Read the model definition and answer for the solid it produces. Units are mm, in the model's axes. A direction names the side the tool comes from. Coordinates: 2 decimals unless noted, no trailing zeros. Order: outer loops, then holes, each group sorted by start corner. A loop starts at its lowest first (then second) coordinate and runs counter-clockwise, first axis right, second up. Notation, with made-up numbers: M 50,57.25 L 83,57.25 A19 cw 83,80.25 Z; hole C 89.5,-27.5 d8. An arc over 180 degrees is marked long. Use a Markdown table: item, result. Add a question column.
1) Each of these flat-tipped pins is pushed along its axis until it touches: pin 1 Ø1 at (y, z) = (100, -25) entering from -X; pin 2 Ø0.9 at (x, y) = (9.5, 155.5) entering from +Z; pin 3 Ø5.5 at (x, y) = (143, 67) entering from +Z; pin 4 Ø2.5 at (x, y) = (149.5, 4) entering from -Z. Where does it stop, or does it pass through?
2) Find section A-A on x = 69.5. Write down the section's boundary in (y, z).
3) Find section B-B on y = 98. Write down the section's boundary in (x, z), plus the area to 3 significant figures.
4) For faces 4 (the face through (153.006, 153, -7)), 5 (the face through (151, 5, -13)), 6 (the face through (10.37, 78, -6)), 7 (the face through (5, 124, -3.5)), determine the directions among +Z, -Z, +X, -X, +Y, -Y from which every point of the face is accessible in a straight line to the end or side of a thin tool.
5) Find section C-C on z = -27.25. Write down the section's boundary in (x, y).
6) Find the intervals of material crossed by probe 1 along Y at (x, z) = (49, -3); probe 2 along Y at (x, z) = (3.75, -2.15) (3 decimals); probe 3 along X at (y, z) = (155, -1.8), in increasing order. Write a range as [from, to].
7) The mould has two halves that part along Y. Classify faces 1 (the face through (81, 148.38, -6)), 2 (the face through (2.406, 2.281, -7.768)), 3 (the face through (153.006, 5, -7)): released by +Y, released by -Y, zero draft, split by the parting line, or undercut.
from build123d import *

# Parameters (mm, degrees)
EXTRUDE_1_DEPTH      = 30
SKETCH_2_R           = 1.5
CUT_EXTRUDE_1_DEPTH  = 5
CUT_EXTRUDE_4_DEPTH  = 307
SKETCH_3_W           = 285.26
SKETCH_3_H           = 138.01
CUT_EXTRUDE_5_DEPTH  = 13
SKETCH_12_W          = 40
SKETCH_12_H          = 50
CUT_EXTRUDE_7_DEPTH  = 3
CUT_EXTRUDE_7_DRAFT  = -30
SKETCH_9_W           = 100
SKETCH_9_H           = 80
CUT_EXTRUDE_8_DEPTH  = 3
CUT_EXTRUDE_8_DRAFT  = -30
CUT_EXTRUDE_9_DEPTH  = 11
FILLET_1_R           = 2
CUT_EXTRUDE_10_DEPTH = 11
FILLET_2_R           = 2
FILLET_3_R           = 2
FILLET_4_R           = 2
CUT_EXTRUDE_11_DEPTH = 5


with BuildPart() as part:
    # Model → 凸台-拉伸1 (new body)
    with BuildSketch(Plane.XY):
        with BuildLine():
            Line((0, 11), (0, 150.75))
            ThreePointArc((0, 150.75), (2.343145751, 156.406854249), (8, 158.75))
            Line((8, 158.75), (298.011203897, 158.75))
            ThreePointArc((298.011203897, 158.75), (303.664092807, 156.410816811), (306.011196041, 150.761211743))
            Line((306.011196041, 150.761211743), (306.207051361, 11.011211743))
            Line((306.207051361, 11.011211743), (306.207051361, 8))
            ThreePointArc((306.207051361, 8), (303.863905611, 2.343145751), (298.207051361, 0))
            Line((298.207051361, 0), (8, 0))
            ThreePointArc((8, 0), (2.343145751, 2.343145751), (0, 8))
            Line((0, 8), (0, 11))
        make_face()
    extrude(amount=-EXTRUDE_1_DEPTH)

    # 草图2 → 切除-拉伸1 (cut)
    with BuildSketch(Plane.XY):
        with Locations((105.108569936, 3.75)):
            Circle(SKETCH_2_R)
        with Locations((9.108569936, 3.75)):
            Circle(SKETCH_2_R)
        with Locations((201.10846029, 3.817270412)):
            Circle(SKETCH_2_R)
        with Locations((297.108366012, 3.951811323)):
            Circle(SKETCH_2_R)
        with Locations((105.108569936, 155)):
            Circle(SKETCH_2_R)
        with Locations((9.108569936, 155)):
            Circle(SKETCH_2_R)
        with Locations((201.10846029, 154.932729588)):
            Circle(SKETCH_2_R)
        with Locations((297.108366012, 154.798188677)):
            Circle(SKETCH_2_R)
        with Locations((3.75, 109.375)):
            Circle(SKETCH_2_R)
        with Locations((3.75, 49.375)):
            Circle(SKETCH_2_R)
        with Locations((302.318900647, 109.584217456)):
            Circle(SKETCH_2_R)
        with Locations((302.402988717, 49.58427638)):
            Circle(SKETCH_2_R)
    extrude(amount=-CUT_EXTRUDE_1_DEPTH, mode=Mode.SUBTRACT)

    # 草图6 → 切除-拉伸4 (cut)
    with BuildSketch(Plane.ZY):
        Polygon((-30, 158.75), (-30, 0), (-15, 0), align=None)
    extrude(amount=-CUT_EXTRUDE_4_DEPTH, mode=Mode.SUBTRACT)

    # 草图3 → 切除-拉伸5 (cut)
    with BuildSketch(Plane.XY):
        with Locations((153, 79.375)):
            Rectangle(SKETCH_3_W, SKETCH_3_H)
    extrude(amount=-CUT_EXTRUDE_5_DEPTH, mode=Mode.SUBTRACT)


with BuildPart() as cut_extrude_7_tool:
    # 草图12 → 切除-拉伸7 (with draft: the straight prism first)
    with BuildSketch(Plane.XY.offset(-13)):
        with Locations((153, 70.37)):
            Rectangle(SKETCH_12_W, SKETCH_12_H)
    extrude(amount=-CUT_EXTRUDE_7_DEPTH)
    # 切除-拉伸7: the draft: its side faces are tilted about the plane it starts from
    cut_extrude_7_sides = [cut_extrude_7_tool.faces().sort_by_distance(p)[0] for p in [
        (153, 45.37, -14.5),
        (173, 70.37, -14.5),
        (153, 95.37, -14.5),
        (133, 70.37, -14.5),
    ]]
    draft(cut_extrude_7_sides, Plane.XY.offset(-13), CUT_EXTRUDE_7_DRAFT)


with BuildPart() as part_1:
    add(part.part)

    # 切除-拉伸7: cut by cut_extrude_7_tool
    add(cut_extrude_7_tool.part, mode=Mode.SUBTRACT)


with BuildPart() as cut_extrude_8_tool:
    # 草图9 → 切除-拉伸8 (with draft: the straight prism first)
    with BuildSketch(Plane.XY.offset(-13)):
        with Locations((75.37, 88.38)):
            Rectangle(SKETCH_9_W, SKETCH_9_H)
    extrude(amount=-CUT_EXTRUDE_8_DEPTH)
    # 切除-拉伸8: the draft: its side faces are tilted about the plane it starts from
    cut_extrude_8_sides = [cut_extrude_8_tool.faces().sort_by_distance(p)[0] for p in [
        (25.37, 88.38, -14.5),
        (75.37, 48.38, -14.5),
        (125.37, 88.38, -14.5),
        (75.37, 128.38, -14.5),
    ]]
    draft(cut_extrude_8_sides, Plane.XY.offset(-13), CUT_EXTRUDE_8_DRAFT)


with BuildPart() as part_2:
    add(part_1.part)

    # 切除-拉伸8: cut by cut_extrude_8_tool
    add(cut_extrude_8_tool.part, mode=Mode.SUBTRACT)

    # 草图14 → 切除-拉伸9 (cut)
    with BuildSketch(Plane.ZY):
        with BuildLine():
            Line((-5.9, 129.38), (-6.1, 129.38))
            ThreePointArc((-6.1, 129.38), (-7.797056275, 128.677056275), (-8.5, 126.98))
            Line((-8.5, 126.98), (-8.5, 120.78))
            ThreePointArc((-8.5, 120.78), (-7.797056275, 119.082943725), (-6.1, 118.38))
            Line((-6.1, 118.38), (-5.9, 118.38))
            ThreePointArc((-5.9, 118.38), (-4.202943725, 119.082943725), (-3.5, 120.78))
            Line((-3.5, 120.78), (-3.5, 126.98))
            ThreePointArc((-3.5, 126.98), (-4.202943725, 128.677056275), (-5.9, 129.38))
        make_face()
    extrude(amount=-CUT_EXTRUDE_9_DEPTH, mode=Mode.SUBTRACT)

    # 圆角1
    fillet_1_edges = [part_2.edges().sort_by_distance(p)[0] for p in [
        (0, 123.88, -3.5),
        (0, 118.38, -6),
        (0, 119.082943725, -7.797056275),
        (0, 128.677056275, -7.797056275),
        (0, 128.677056275, -4.202943725),
        (0, 129.38, -6),
        (0, 123.88, -8.5),
        (0, 119.082943725, -4.202943725),
    ]]
    fillet(fillet_1_edges, radius=FILLET_1_R)

    # 草图15 → 切除-拉伸10 (cut)
    with BuildSketch(Plane.XZ):
        with BuildLine():
            Line((222.53, -3.959687417), (229.73, -3.959687417))
            ThreePointArc((229.73, -3.959687417), (231.427056275, -4.662631142), (232.13, -6.359687417))
            Line((232.13, -6.359687417), (232.13, -6.559687417))
            ThreePointArc((232.13, -6.559687417), (231.427056275, -8.256743692), (229.73, -8.959687417))
            Line((229.73, -8.959687417), (222.53, -8.959687417))
            ThreePointArc((222.53, -8.959687417), (220.832943725, -8.256743692), (220.13, -6.559687417))
            Line((220.13, -6.559687417), (220.13, -6.359687417))
            ThreePointArc((220.13, -6.359687417), (220.832943725, -4.662631142), (222.53, -3.959687417))
        make_face()
    extrude(amount=-CUT_EXTRUDE_10_DEPTH, mode=Mode.SUBTRACT)

    # 圆角2
    fillet_2_edges = [part_2.edges().sort_by_distance(p)[0] for p in [
        (226.13, 0, -3.959687417),
        (232.13, 0, -6.459687417),
        (231.427056275, 0, -8.256743692),
        (220.832943725, 0, -4.662631142),
        (220.13, 0, -6.459687417),
        (220.832943725, 0, -8.256743692),
        (226.13, 0, -8.959687417),
        (231.427056275, 0, -4.662631142),
    ]]
    fillet(fillet_2_edges, radius=FILLET_2_R)

    # 圆角3
    fillet_3_edges = [part_2.edges().sort_by_distance(p)[0] for p in [
        (10.37, 129.38, -6),
        (10.37, 128.677056275, -7.797056275),
        (10.37, 123.88, -8.5),
        (10.37, 119.082943725, -7.797056275),
        (10.37, 118.38, -6),
        (10.37, 119.082943725, -4.202943725),
        (10.37, 123.88, -3.5),
        (10.37, 128.677056275, -4.202943725),
    ]]
    fillet(fillet_3_edges, radius=FILLET_3_R)

    # 圆角4
    fillet_4_edges = [part_2.edges().sort_by_distance(p)[0] for p in [
        (220.13, 10.37, -6.459687417),
        (220.832943725, 10.37, -8.256743692),
        (226.13, 10.37, -8.959687417),
        (231.427056275, 10.37, -8.256743692),
        (232.13, 10.37, -6.459687417),
        (231.427056275, 10.37, -4.662631142),
        (226.13, 10.37, -3.959687417),
        (220.832943725, 10.37, -4.662631142),
    ]]
    fillet(fillet_4_edges, radius=FILLET_4_R)


with BuildPart() as body_2:
    # Split Bodies 1: the piece on the far side of the plane
    add(part_2.part)
    split(bisect_by=Plane(origin=(153.005601949, 0, 0), x_dir=(0, 0, 1), z_dir=(1, 0, 0)), keep=Keep.BOTTOM)

    # 草图19 → 切除-拉伸11 (cut)
    with BuildSketch(Plane(origin=(153.005601949, 0, 0), x_dir=(0, 0, -1), z_dir=(1, 0, 0))):
        Polygon((13, 148.38), (13, 95.37), (16, 93.637949192), (24.011338583, 95.37), (30, 158.75), (13, 158.75), align=None)
        Polygon((19.286929134, 45.37), (15, 0), (13, 0), (13, 45.37), (16, 47.102050808), align=None)
    extrude(amount=-CUT_EXTRUDE_11_DEPTH, mode=Mode.SUBTRACT)


with BuildPart() as part_3:
    add(part_2.part)

    # Split Bodies 1
    split(bisect_by=Plane(origin=(153.005601949, 0, 0), x_dir=(0, 0, 1), z_dir=(1, 0, 0)), keep=Keep.TOP)


solid = body_2.part
Check result:
| question | item | result |
|---|---|---|
| 1 | pin 1 | passes through |
| 1 | pin 2 | stops at z = -5 |
| 1 | pin 3 | stops at z = -16 |
| 1 | pin 4 | stops at z = -13 |
| 2 | outline | M 0,-15 L 158.75,-30 L 158.75,0 L 148.38,0 L 148.38,-13 L 128.38,-13 L 126.65,-16 L 50.11,-16 L 48.38,-13 L 10.37,-13 L 10.37,0 L 0,0 Z |
| 3 | outline | M 0,-24.26 L 148.01,-24.26 L 148.01,-13 L 125.37,-13 L 123.64,-16 L 27.1,-16 L 25.37,-13 L 10.37,-13 L 10.37,0 L 0,0 Z |
| 3 | area | 1,510 mm2 |
| 4 | face 4 | +Z, -Z, +X, +Y, -Y |
| 4 | face 5 | -Z, +X, +Y, -Y |
| 4 | face 6 | +Z, +X |
| 4 | face 7 | +X, -X |
| 5 | outline | M 0,129.65 L 148.01,129.65 L 148.01,158.75 L 8,158.75 A8 ccw 0,150.75 Z |
| 6 | probe 1 | y = [0, 10.37], [148.38, 158.75] |
| 6 | probe 2 | y = [1.222, 47.875], [50.875, 107.875], [110.875, 157.528] |
| 6 | probe 3 | x = [1.22, 7.61], [10.61, 103.61], [106.61, 153.01] |
| 7 | face 1 | undercut |
| 7 | face 2 | released by -Y |
| 7 | face 3 | zero draft |
